Can you work these out from the model? Positions are in its coordinate system, mm. Face numbers are marked on the shaded views. A direction names the side the tool comes from. Give positions to 0.01 mm unless a question says otherwise; leave off trailing zeros. Order: outer loops, then holes, each group sorted by start corner. A loop starts at its lowest first (then second) coordinate and runs counter-clockwise, first axis right, second up. Notation, with made-up numbers: M -4,54 L 38,54 A34 cw 38,93 Z; hole C 19,50.25 d3. An arc over 180 degrees is marked long. Write each question's results on one line, items separated by ' | '.
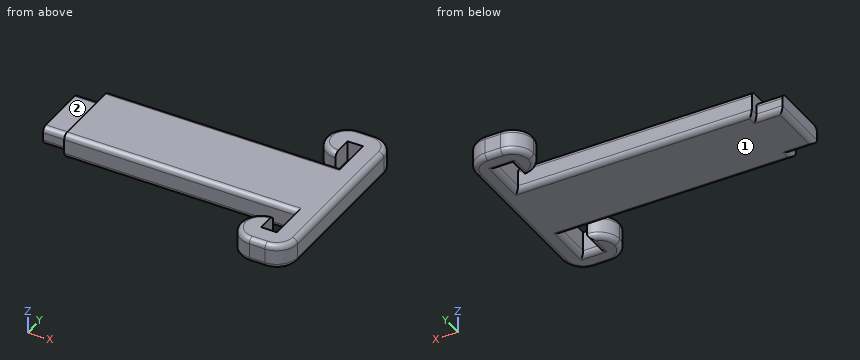
from build123d import *

# Parameters (mm, degrees)
F1_DEPTH = 4.75
F0_W     = 5
F0_H     = 11.6
F2_DEPTH = 3.5
F3_R     = 1


with BuildPart() as f1:
    # F0 (on Top) → F1 (new body)
    with BuildSketch(Plane.XY):
        with BuildLine():
            Line((-45, 7.4), (-45, 5.8))
            Line((-45, 5.8), (-45, -5.8))
            Line((-45, -5.8), (-45, -7.4))
            Line((-45, -7.4), (0, -7.4))
            Line((0, -7.4), (0, -14.5))
            Line((0, -14.5), (-3, -14.5))
            Line((-3, -14.5), (-3, -10.5))
            ThreePointArc((-3, -10.5), (-5.828427, -11.671573), (-7, -14.5))
            ThreePointArc((-7, -14.5), (-5.828427, -17.328427), (-3, -18.5))
            Line((-3, -18.5), (0, -18.5))
            ThreePointArc((0, -18.5), (2.828427, -17.328427), (4, -14.5))
            Line((4, -14.5), (4, 0))
            Line((4, 0), (4, 14.5))
            ThreePointArc((4, 14.5), (2.828427, 17.328427), (0, 18.5))
            Line((0, 18.5), (-3, 18.5))
            ThreePointArc((-3, 18.5), (-5.828427, 17.328427), (-7, 14.5))
            ThreePointArc((-7, 14.5), (-5.828427, 11.671573), (-3, 10.5))
            Line((-3, 10.5), (-3, 14.5))
            Line((-3, 14.5), (0, 14.5))
            Line((0, 14.5), (0, 7.4))
            Line((0, 7.4), (-45, 7.4))
        make_face()
    extrude(amount=F1_DEPTH)

    # F0 (on Top) → F2 (join)
    with BuildSketch(Plane.XY):
        with Locations((-47.5, 0)):
            Rectangle(F0_W, F0_H)
    extrude(amount=F2_DEPTH)

    # F3
    f3_edges = [f1.edges().sort_by_distance(p)[0] for p in [
        (-47.5, -5.8, 3.5),
        (-47.5, 5.8, 3.5),
        (-22.5, -7.4, 4.75),
        (-22.5, 7.4, 4.75),
        (-7, 14.5, 4.75),
        (2.828427, 17.328427, 0),
        (-1.5, 18.5, 0),
        (-7, 14.5, 0),
        (-3, 12.5, 0),
        (-1.5, 14.5, 0),
        (0, 10.95, 0),
        (-22.5, 7.4, 0),
        (-45, 6.6, 0),
        (-47.5, 5.8, 0),
        (-50, 0, 0),
        (-47.5, -5.8, 0),
        (-45, -6.6, 0),
        (-22.5, -7.4, 0),
        (0, -10.95, 0),
        (-1.5, -14.5, 0),
        (-3, -12.5, 0),
        (-7, -14.5, 0),
        (-1.5, -18.5, 0),
        (2.828427, -17.328427, 0),
        (4, 0, 0),
    ]]
    fillet(f3_edges, radius=F3_R)


solid = f1.part
(1) Will these pins go through, and if not, where does the flat tip stop? P1, Ø0.8, axis at x = -47.5, z = 2, coming from the +Y side; P2, Ø1.2, axis at x = -48.5, z = 1.5, coming from the -Y side; P3, Ø2.5, axis at x = -47.5, y = 2, coming from the +Z side.
Data:
P1: stops at y = 5.8 | P2: stops at y = -5.8 | P3: stops at z = 3.5
(2) Imagine slicing it at C-C, the plane x = -39.5. Write out the boundary of the cut face in (y, z).
Data:
outline: M -7.4,1 A1 ccw -6.4,0 L 6.4,0 A1 ccw 7.4,1 L 7.4,3.75 A1 ccw 6.4,4.75 L -6.4,4.75 A1 ccw -7.4,3.75 Z
(3) Imagine slicing it at D-D, the plane y = 2. Write out the boundary of the cut face in (x, z).
Data:
outline: M -50,1 A1 ccw -49,0 L 3,0 A1 ccw 4,1 L 4,3.75 A1 ccw 3,4.75 L -45,4.75 L -45,3.5 L -50,3.5 Z
(4) For the marked faces 1 and 2, which set-ups out of +Z, -Z, +X, -X, +Y, -Y let a thin tool reach every point of the face, with its end or its side?
Data:
face 1: -Z, +X, -X, +Y, -Y | face 2: +Z, -X, +Y, -Y
(5) Imagine slicing it at B-B, the plane z = 1.7. Write out the boundary of the cut face in (x, y).
Data:
outline: M -50,-5.8 L -45,-5.8 L -45,-7.4 L 0,-7.4 L 0,-14.5 L -3,-14.5 L -3,-10.5 A4 ccw -3,-18.5 L 0,-18.5 A4 ccw 4,-14.5 L 4,14.5 A4 ccw 0,18.5 L -3,18.5 A4 ccw -3,10.5 L -3,14.5 L 0,14.5 L 0,7.4 L -45,7.4 L -45,5.8 L -50,5.8 Z
(6) I need wall thicknesses on L1, parallel to Y at x = -5, z = 0.2; L2, parallel to Y at x = -42.5, z = 2.6; L3, parallel to Y at x = -6, z = 2.9. Which ranges of each line are inside material? Lowest first, please. Write a range as from..to.
Data:
L1: y = -17.49..-11.51, -7..7, 11.51..17.49 | L2: y = -7.4..7.4 | L3: y = -17.15..-11.85, -7.4..7.4, 11.85..17.15
(7) Imagine slicing it at A-A, the plane y = 9. Write out the boundary of the cut face in (x, z).
Data:
outline: M 0,1 A1 ccw 1,0 L 3,0 A1 ccw 4,1 L 4,3.75 A1 ccw 3,4.75 L 0,4.75 Z
